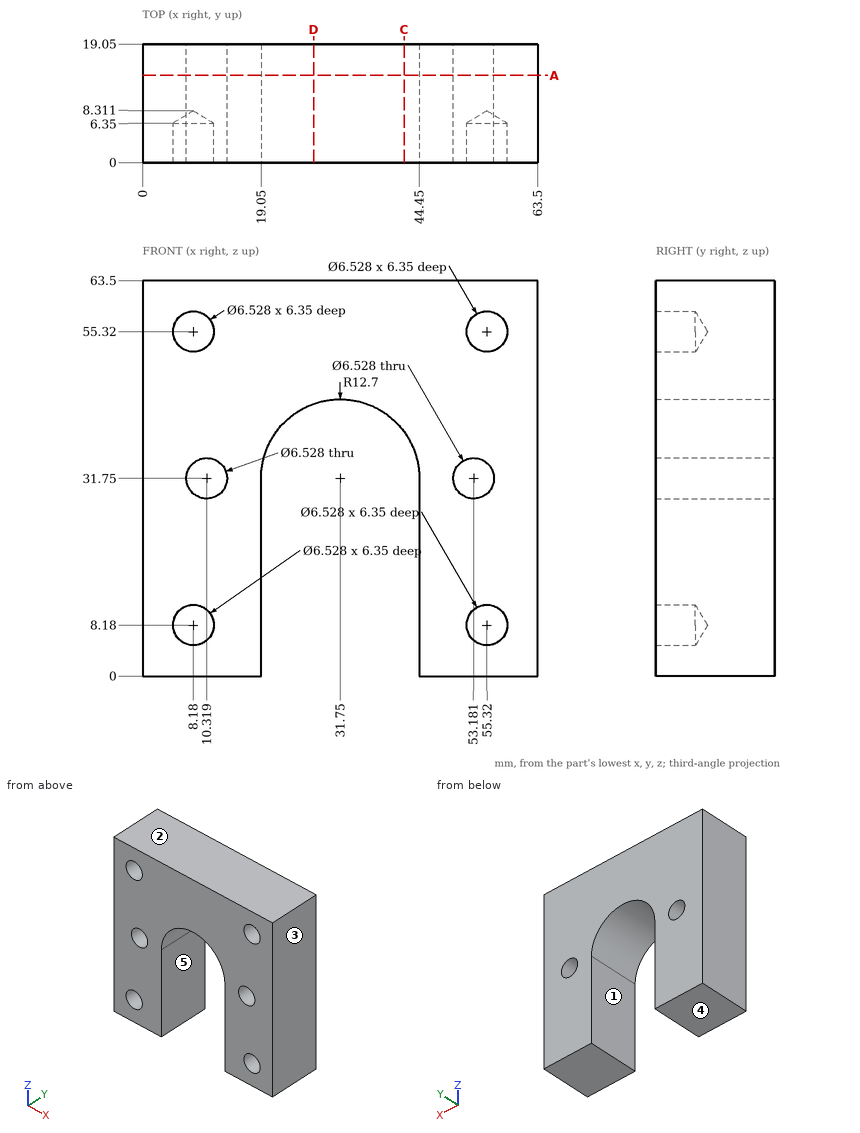
The drawing under review shows one solid part. Ordinate dimensions are in mm from its lowest x, y, z. A direction names the side the tool comes from. Round coordinates to 2 decimals unless told otherwise and drop trailing zeros. Write each loop counter-clockwise with the first axis right and the second up, starting at its lowest first coordinate (ties: lowest second). Pieces come first, ordered by that corner, then holes.
(1) Wall thickness on L1, parallel to X at y = 5, z = 8.18; L2, parallel to X at y = 2.75, z = 55.32; L3, parallel to X at y = 13, z = 8: over which ranges is each line inside the solid? List them lowest first.
(2) We need section C-C on x = 42. Give the boundary of the cut face in (y, z), and give its area (3 significant figures).
(3) We need section D-D on x = 27.5. Give the boundary of the cut face in (y, z), and give its area (3 significant figures).
(4) We need section A-A on y = 14. Give the number of separate pieces and of enclosed holes in the cut face, and give its area (3 significant figures).
(5) Machinability: for the marked faces 1 and 2, which of the approach directions +Z, -Z, +X, -X, +Y, -Y give a long, thin tool a straight path to every point of the face, cutting with its end or side? Answer none if there is none.
(6) Insertion check: pin 1 (7.5 mm diameter, centred on x = 10.32, z = 31.75, fed in from +Y); pin 2 (5 mm diameter, centred on x = 55.32, z = 55.32, fed in from -Y); pin 3 (1.5 mm diameter, centred on x = 42.5, z = 8.5, fed in from +Y) (3 decimals); pin 4 (6 mm diameter, centred on x = 8.18, z = 55.32, fed in from -Y). Each pin has a flat end and moves straight along its axis. Give the tip position at first contact, or say it passes through.
(7) Mouldability with a two-part tool opening along X and no side actions: class the marked faces 3, 4 and 5 as +X half, -X half, draft (parallel to the pull), parting line (faces both ways), or undercut.
Findings below:
1. L1: x = 0 to 4.92, 11.44 to 19.05, 44.45 to 52.06, 58.58 to 63.5
1. L2: x = 0 to 4.92, 11.44 to 52.06, 58.58 to 63.5
1. L3: x = 0 to 19.05, 44.45 to 63.5
2. outline: (0, 39.25) - (19.05, 39.25) - (19.05, 63.5) - (0, 63.5) - close
2. area: 462 mm2
3. outline: (0, 43.72) - (19.05, 43.72) - (19.05, 63.5) - (0, 63.5) - close
3. area: 377 mm2
4. separate pieces: 1
4. enclosed holes: 2
4. area: 2,910 mm2
5. face 1: -Z, +Y, -Y
5. face 2: +Z, +X, -X, +Y, -Y
6. pin 1: stops at y = 19.05
6. pin 2: stops at y = 6.81
6. pin 3: passes through
6. pin 4: stops at y = 6.51
7. face 3: +X half
7. face 4: draft
7. face 5: undercut
